Can you work these out from the drawing? Everything is in mm from the part's minimum corner. A direction names the side the tool comes from. Round coordinates to 2 decimals unless told otherwise and drop trailing zeros. Loops run counter-clockwise (first coordinate to the right, second up) from the corner with the lowest first, then second, coordinate; pieces in that order, holes last. Notation, with made-up numbers: (2.25, 52) -> (45.25, 52) arc R21 cw to (45.25, 76) -> close; hole circle Ø11 at (-6, 46). An arc over 180 degrees is marked (long way). Answer as a JSON object with one key per item and string values.
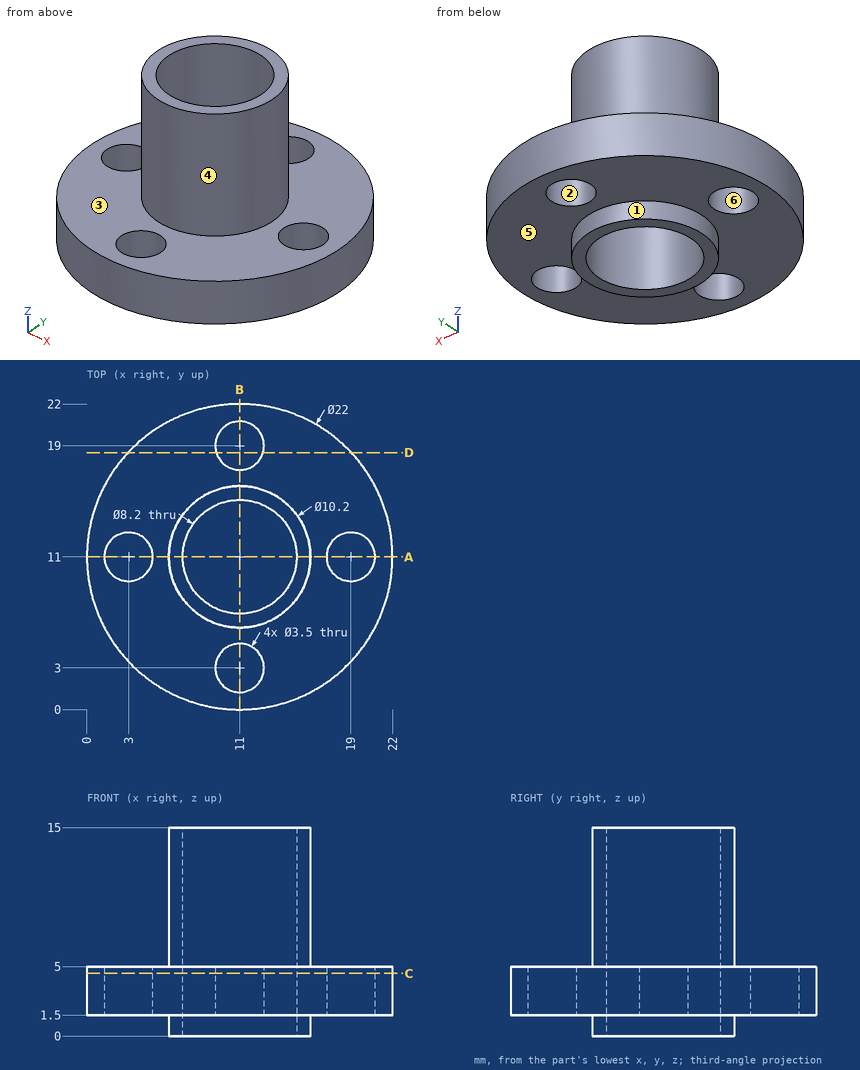
Q1. I'm going to push flat-ended pins straight in: pin 1 (4 mm diameter, centred on x = 3, y = 11, fed in from +Z); pin 2 (6.5 mm diameter, centred on x = 7.5, y = 7, fed in from +Z); pin 3 (6.5 mm diameter, centred on x = 11, y = 11, fed in from -Z); pin 4 (1.5 mm diameter, centred on y = 12, z = 12, fed in from -X). Where does each tip first touch, or does it pass through?
Determined:
{"pin 1": "z = 5", "pin 2": "z = 15", "pin 3": "through", "pin 4": "x = 5.91"}
Q2. I want a section at D-D, the plane y = 18.5. Write out the boundary of the cut face in (x, z), then the cut area to 3 significant figures.
Determined:
{"outline": "(2.95, 1.5) -> (9.32, 1.5) -> (9.32, 5) -> (2.95, 5) -> close; (12.68, 1.5) -> (19.05, 1.5) -> (19.05, 5) -> (12.68, 5) -> close", "area": "44.6 mm²"}
Q3. We'd pull the mould along Y, two halves only. Please class the marked faces 1, 2 and 3: pulls with the +Y half, pulls with the -Y half, needs draft (parallel to the pull), parting line crosses it, or undercut.
Determined:
{"face 1": "parting line crosses it", "face 2": "undercut", "face 3": "needs draft"}
Q4. I want a section at A-A, the plane y = 11. Write out the boundary of the cut face in (x, z), then the cut area to 3 significant figures.
Determined:
{"outline": "(0, 1.5) -> (1.25, 1.5) -> (1.25, 5) -> (0, 5) -> close; (4.75, 1.5) -> (5.9, 1.5) -> (5.9, 0) -> (6.9, 0) -> (6.9, 15) -> (5.9, 15) -> (5.9, 5) -> (4.75, 5) -> close; (15.1, 0) -> (16.1, 0) -> (16.1, 1.5) -> (17.25, 1.5) -> (17.25, 5) -> (16.1, 5) -> (16.1, 15) -> (15.1, 15) -> close; (20.75, 1.5) -> (22, 1.5) -> (22, 5) -> (20.75, 5) -> close", "area": "46.8 mm²"}
Q5. I want a section at C-C, the plane z = 4.5. Write out the boundary of the cut face in (x, y).
Determined:
{"outline": "circle Ø22 at (11, 11); hole circle Ø3.5 at (3, 11); hole circle Ø8.2 at (11, 11); hole circle Ø3.5 at (11, 3); hole circle Ø3.5 at (11, 19); hole circle Ø3.5 at (19, 11)"}
Q6. If I drill on L1, parallel to Y at x = 11, z = 2.45; L2, parallel to X at y = 10.75, z = 7; L3, parallel to Y at x = 11, z = 9.25, over which ranges is the centre line in solid material (lowest first)? Write a range as [from, to].
Determined:
{"L1": "[0, 1.25], [4.75, 6.9], [15.1, 17.25], [20.75, 22]", "L2": "[5.91, 6.91], [15.09, 16.09]", "L3": "[5.9, 6.9], [15.1, 16.1]"}
Q7. On a 3-axis mill with a long thin cutter (end or side, diameter ignored), from which of +Z, -Z, +X, -X, +Y, -Y can I reach the whole of each face in a straight line? I mean the marked faces 4, 5 and 6. Say none if no direction works.
Determined:
{"face 4": "+Z", "face 5": "-Z", "face 6": "+Z, -Z"}
